Check sheet for the modelled part. Datum: model origin and axes. Units: mm. Face numbers are marked on the shaded views. Give positions to 0.01 mm unless a question says otherwise; leave off trailing zeros. Loops run counter-clockwise (first coordinate to the right, second up) from the corner with the lowest first, then second, coordinate; pieces in that order, holes last. Notation, with made-up numbers: (31, 50) - (76, 50) arc R23 ccw to (76, 77) - close; hole circle Ø5 at (-3.75, 56). An arc over 180 degrees is marked (long way). Answer in a Markdown table with one row per item. Add a question column.
(1) Sectioned sample at A-A on y = 2.5. Enter the section's corners in (x, z).
(2) Sectioned sample at D-D on y = 1.25. Enter the section's corners in (x, z), then the cut area to 3 significant figures.
(3) Thickness scan on L1, parallel to Z at x = -4.5, y = 2.75; L2, parallel to Z at x = -6, y = 6.25; L3, parallel to Z at x = 8, y = 1.25. Record the ranges inside material, lowest first.
(4) Sectioned sample at B-B on z = -4.75. Enter the section's corners in (x, y).
(5) Go/stop test with flat-tipped pins: P1, Ø0.7, axis at y = 7, z = 0, coming from the -X side; P2, Ø0.7, axis at x = -8, y = 5.5, coming from the +Z side; P3, Ø0.5, axis at y = 5.5, z = -0.5, coming from the +X side. Record where each tip stops, or that it passes through.
(6) Sectioned sample at C-C on x = 12.75. Enter the section's corners in (y, z), then the cut area to 3 significant figures.
(7) Draft check along Y on the marked faces 1, 2 and 3. Enter one of: released by +Y, released by -Y, zero draft, split by the parting line, or undercut.
from build123d import *

# Parameters (mm, degrees)
SKETCH_1_W           = 30
SKETCH_1_H           = 15
EXTRUDE_1_DEPTH      = 5
CUT_EXTRUDE_1_REACH  = 33.325
FILLET_1_R           = 0.2
SKETCH_3_W           = 3
SKETCH_3_H           = 3
EXTRUDE_2_DEPTH      = 1
EXTRUDE_3_DEPTH      = 2
EXTRUDE_3_DEPTH_BACK = 2
CUT_EXTRUDE_2_REACH  = 28.652
FILLET_2_R           = 0.1


with BuildPart() as part:
    # 草图1 → 凸台-拉伸1 (new body)
    with BuildSketch(Plane(origin=(0, 0, 0), x_dir=(1, 0, 0), z_dir=(0, 1, 0))):
        Rectangle(SKETCH_1_W, SKETCH_1_H)
    extrude(amount=EXTRUDE_1_DEPTH)

    # 草图2 → 切除-拉伸1 (cut, up to next)
    with BuildSketch(Plane.ZY.offset(15), mode=Mode.PRIVATE) as cut_extrude_1_sk1:
        with BuildLine():
            Line((-1.5, 0), (-1.5, 0.677124344))
            ThreePointArc((-1.5, 0.677124344), (-1.780042303, 1.088161527), (-1.95, 1.555590279))
            Line((-1.95, 1.555590279), (-1.95, 2.8))
            Line((-1.95, 2.8), (1.95, 2.8))
            Line((1.95, 2.8), (1.95, 1.555590279))
            ThreePointArc((1.95, 1.555590279), (1.780042303, 1.088161527), (1.5, 0.677124344))
            Line((1.5, 0.677124344), (1.5, 0))
            Line((1.5, 0), (-1.5, 0))
        make_face()
    cut_extrude_1_tool1 = extrude(cut_extrude_1_sk1.sketch, amount=-CUT_EXTRUDE_1_REACH, mode=Mode.PRIVATE) & part.part
    add(cut_extrude_1_tool1.solids().sort_by_distance((-15, 1.479302, 0))[0], mode=Mode.SUBTRACT)

    # 圆角1
    fillet_1_edges = [part.edges().sort_by_distance(p)[0] for p in [
        (15, 2.5, -7.5),
        (-15, 2.5, -7.5),
        (0, 0, -7.5),
        (-15, 0, -4.5),
        (0, 0, -1.5),
        (-15, 2.5, 7.5),
        (15, 2.5, 7.5),
        (0, 0, 7.5),
        (0, 5, -7.5),
        (15, 5, 0),
        (0, 5, 7.5),
        (-15, 5, 0),
        (15, 0, -4.5),
    ]]
    fillet(fillet_1_edges, radius=FILLET_1_R)

    # 草图3 → 凸台-拉伸2 (add)
    with BuildSketch(Plane(origin=(0, 5, 0), x_dir=(-1, 0, 0), z_dir=(0, 1, 0))):
        with Locations((7.5, 0)):
            Rectangle(SKETCH_3_W, SKETCH_3_H)
    extrude(amount=EXTRUDE_2_DEPTH)

    # 草图4 → 凸台-拉伸3 (add, two sides: drawn at the far end of the back side and taken through both)
    with BuildSketch(Plane.XY.offset(-EXTRUDE_3_DEPTH_BACK)):
        with BuildLine():
            Line((-9.45, 7.5), (-5.55, 7.5))
            Line((-5.55, 7.5), (-5.55, 6.555590279))
            ThreePointArc((-5.55, 6.555590279), (-5.719957697, 6.088161527), (-6, 5.677124344))
            Line((-6, 5.677124344), (-9, 5.677124344))
            ThreePointArc((-9, 5.677124344), (-9.280042303, 6.088161527), (-9.45, 6.555590279))
            Line((-9.45, 6.555590279), (-9.45, 7.5))
        make_face()
    extrude(amount=EXTRUDE_3_DEPTH + EXTRUDE_3_DEPTH_BACK)

    # 草图5 → 切除-拉伸2 (cut, up to next)
    with BuildSketch(Plane.ZY.offset(9.45), mode=Mode.PRIVATE) as cut_extrude_2_sk1:
        with BuildLine():
            Line((-1.95, 7.5), (-1.95, 6.555590279))
            ThreePointArc((-1.95, 6.555590279), (-1.780042303, 6.088161527), (-1.5, 5.677124344))
            Line((-1.5, 5.677124344), (-2, 5.677124344))
            Line((-2, 5.677124344), (-2, 7.5))
            Line((-2, 7.5), (-1.95, 7.5))
        make_face()
    cut_extrude_2_tool1 = extrude(cut_extrude_2_sk1.sketch, amount=-CUT_EXTRUDE_2_REACH, mode=Mode.PRIVATE) & part.part
    # 草图5 → 切除-拉伸2 (cut, up to next)
    with BuildSketch(Plane.ZY.offset(9.45), mode=Mode.PRIVATE) as cut_extrude_2_sk2:
        with BuildLine():
            Line((2, 5.677124344), (2, 7.5))
            Line((2, 7.5), (1.95, 7.5))
            Line((1.95, 7.5), (1.95, 6.555590279))
            ThreePointArc((1.95, 6.555590279), (1.780042303, 6.088161527), (1.5, 5.677124344))
            Line((1.5, 5.677124344), (2, 5.677124344))
        make_face()
    cut_extrude_2_tool2 = extrude(cut_extrude_2_sk2.sketch, amount=-CUT_EXTRUDE_2_REACH, mode=Mode.PRIVATE) & part.part
    add(cut_extrude_2_tool1.solids().sort_by_distance((-9.45, 6.175075, -1.873038))[0], mode=Mode.SUBTRACT)
    add(cut_extrude_2_tool2.solids().sort_by_distance((-9.45, 6.175075, 1.873038))[0], mode=Mode.SUBTRACT)

    # 圆角2
    fillet_2_edges = [part.edges().sort_by_distance(p)[0] for p in [
        (-5.55, 7.5, 0),
        (-9.45, 7.5, 0),
        (-7.5, 7.5, -1.95),
        (-7.5, 7.5, 1.95),
    ]]
    fillet(fillet_2_edges, radius=FILLET_2_R)


solid = part.part
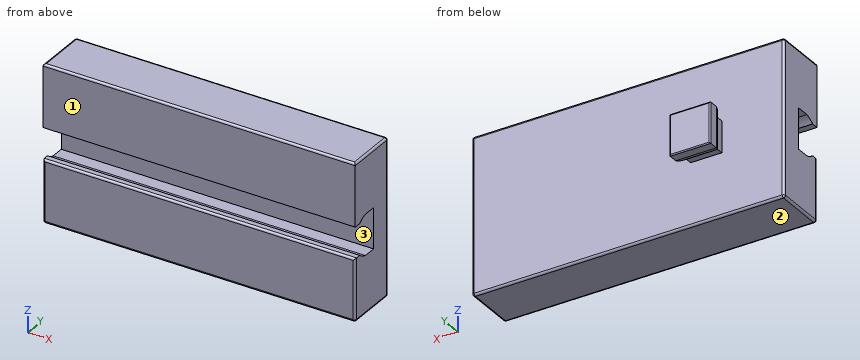
Reply:
| question | item | result |
|---|---|---|
| 1 | outline | (-15, -7.3) arc R0.2 ccw to (-14.8, -7.5) - (14.8, -7.5) arc R0.2 ccw to (15, -7.3) - (15, -1.95) - (-15, -1.95) - close; (-15, 1.95) - (15, 1.95) - (15, 7.3) arc R0.2 ccw to (14.8, 7.5) - (-14.8, 7.5) arc R0.2 ccw to (-15, 7.3) - close |
| 2 | outline | (-15, -7.3) arc R0.2 ccw to (-14.8, -7.5) - (14.8, -7.5) arc R0.2 ccw to (15, -7.3) - (15, -1.85) - (-15, -1.85) - close; (-15, 1.85) - (15, 1.85) - (15, 7.3) arc R0.2 ccw to (14.8, 7.5) - (-14.8, 7.5) arc R0.2 ccw to (-15, 7.3) - close |
| 2 | area | 339 mm^2 |
| 3 | L1 | -7.5 to -1.95, 1.95 to 7.5 |
| 3 | L2 | -1.85 to 1.85 |
| 3 | L3 | -7.5 to -1.85, 1.85 to 7.5 |
| 4 | outline | (-15, 0.2) arc R0.2 ccw to (-14.8, 0) - (14.8, 0) arc R0.2 ccw to (15, 0.2) - (15, 4.8) arc R0.2 ccw to (14.8, 5) - (-14.8, 5) arc R0.2 ccw to (-15, 4.8) - close |
| 5 | P1 | x = -9.45 |
| 5 | P2 | z = 1.64 |
| 5 | P3 | x = -5.94 |
| 6 | outline | (0, -7.3) arc R0.2 ccw to (0.2, -7.5) - (4.8, -7.5) arc R0.2 ccw to (5, -7.3) - (5, 7.3) arc R0.2 ccw to (4.8, 7.5) - (0.2, 7.5) arc R0.2 ccw to (0, 7.3) - (0, 1.5) - (0.68, 1.5) arc R2 cw to (1.56, 1.95) - (2.8, 1.95) - (2.8, -1.95) - (1.56, -1.95) arc R2 cw to (0.68, -1.5) - (0.2, -1.5) arc R0.2 ccw to (0, -1.7) - close |
| 6 | area | 65.0 mm^2 |
| 7 | face 1 | released by -Y |
| 7 | face 2 | zero draft |
| 7 | face 3 | undercut |
